from build123d import *

# Parameters (mm, degrees)
SKETCH1248_R           = 5
OBJ1_DEPTH = 60
CLONE2D015_R           = 3
OBJ2_DEPTH = 17
SKETCH1249_R           = 3
OBJ3 = 17


with BuildPart() as obj1:
    # Sketch1248 (on Sketch) → obj1 (new body, symmetric)
    with BuildSketch(Plane(origin=(471.25, -267, 0), x_dir=(-1, 0, 0), z_dir=(0, 0, 1))):
        Circle(SKETCH1248_R)
    extrude(amount=OBJ1_DEPTH, both=True)


with BuildPart() as obj2:
    # Clone2D015 (on Sketch) → obj2 (new body)
    with BuildSketch(Plane(origin=(471.25, -250, 50), x_dir=(0, 0, 1), z_dir=(0, -1, 0))):
        Circle(CLONE2D015_R)
    extrude(amount=OBJ2_DEPTH)


with BuildPart() as clone002:
    with BuildSketch(Plane(origin=(471.25, -250, -50), x_dir=(0, 0, 1), z_dir=(0, -1, 0))):
        Circle(SKETCH1249_R)
    extrude(amount=OBJ3)

    # Fusion008: union obj1, obj2
    add(obj1.part)
    add(obj2.part)


with BuildPart() as clone002_1:
    # Clone002 placement: moved
    add(clone002.part.moved(Location((0, 0, 920))))


solid = clone002_1.part
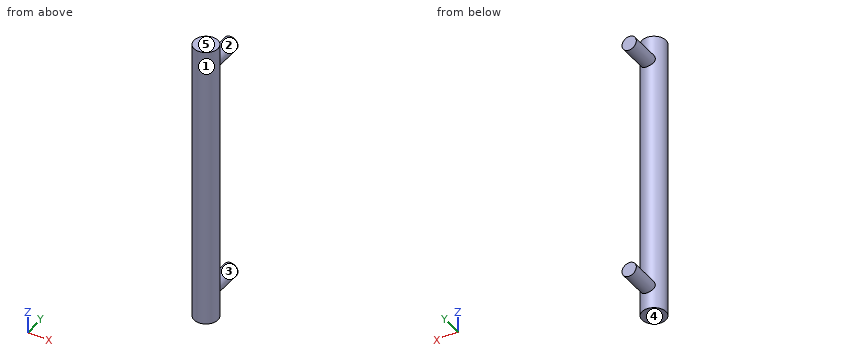
Can you work these out from the model? Positions are in its coordinate system, mm. Face numbers are marked on the shaded views. A direction names the side the tool comes from. Coordinates: 2 decimals unless noted, no trailing zeros. Loops run counter-clockwise (first coordinate to the right, second up) from the corner with the lowest first, then second, coordinate; pieces in that order, holes last. Notation, with made-up numbers: M 76,-29 L 90,-29 A31 ccw 90,9 Z; hole C -30.5,46 d2. An arc over 180 degrees is marked long. Return JSON: item names as keys, results as strings. Group by question number.
Item 1: If I drill on L1, parallel to Z at x = 468.75, y = -252.75; L2, parallel to Z at x = 471.75, y = -258.5; L3, parallel to X at y = -263, z = 916, over which ranges is the centre line in solid material (lowest first)? Write a range as from..to.
Item 2: Imagine slicing it at D-D (z = 893). Please give me the cut outline in (x, y), and give its area (3 significant figures).
Item 3: Imagine slicing it at B-B (y = -260.75). Please give me the cut outline in (x, z), and give its area (3 significant figures).
Item 4: On a 3-axis mill with a long thin cutter (end or side, diameter ignored), from which of +Z, -Z, +X, -X, +Y, -Y can I reach the whole of each face in a straight line? I mean the marked faces 1 and 2. Say none if no direction works.
Item 5: Imagine slicing it at C-C (z = 970). Please give me the cut outline in (x, y).
Item 6: I'm going to push flat-ended pins straight in: pin 1 Ø4 at (x, z) = (468.5, 961) entering from +Y; pin 2 Ø1.5 at (y, z) = (-266, 891) entering from +X. Where does each tip first touch, or does it pass through?
Item 7: Imagine slicing it at A-A (x = 471.25). Please give me the cut outline in (y, z), and give its area (3 significant figures).
Item 8: Thinking about a two-plate mould opening in Z: for the marked faces 3, 4 and 5, which applies, released by +Z, released by -Z, zero draft, split by the parting line, or undercut?
Verdict:
{
 "1": {"L1": "z = 868.34..871.66, 968.34..971.66", "L2": "z = 867.04..872.96, 967.04..972.96", "L3": "x = 468.25..474.25"},
 "2": {"outline": "C 471.25,-267 d10", "area": "78.5 mm^2"},
 "3": {"outline": "C 471.25,870 d6; C 471.25,970 d6", "area": "56.5 mm^2"},
 "4": {"face 1": "none", "face 2": "+Y"},
 "5": {"outline": "M 468.25,-263 A5 ccw long 474.25,-263 L 474.25,-250 L 468.25,-250 Z"},
 "6": {"pin 1": "stops at y = -262.06", "pin 2": "stops at x = 476.24"},
 "7": {"outline": "M -272,860 L -262,860 L -262,867 L -250,867 L -250,873 L -262,873 L -262,967 L -250,967 L -250,973 L -262,973 L -262,980 L -272,980 Z", "area": "1,340 mm^2"},
 "8": {"face 3": "undercut", "face 4": "released by -Z", "face 5": "released by +Z"}
}
